Could you check a few things on this model? Use its own coordinates, in mm. A direction names the side the tool comes from. Coordinates: 2 decimals unless noted, no trailing zeros. Write each loop counter-clockwise with the first axis right and the second up, starting at its lowest first coordinate (ties: lowest second). Pieces come first, ordered by that corner, then holes.
Autodesk Inventor part; units mm, degrees
ref_plane "YZ Plane" through (0, 0, 0) normal (1, 0, 0) x (0, 1, 0)
ref_plane "XZ Plane" through (0, 0, 0) normal (0, 1, 0) x (-1, 0, 0)
ref_plane "XY Plane" through (0, 0, 0) normal (0, 0, 1) x (1, 0, 0)
sketch "Boceto1" plane through (0, 0, 0) normal (0, 0, 1) x (1, 0, 0)
  line L0 (-350, 205) -> (350, 205)
  line L1 (350, 205) -> (350, -205)
  line L2 (350, -205) -> (-350, -205)
  line L3 (-350, -205) -> (-350, 205)
  line L4 (-350, 205) -> (350, -205) construction
  line L5 (350, 205) -> (-350, -205) construction
  point P0 (0, 0)
  dimension "d0" = 700
  dimension "d1" = 410
extrude "Placa1" add sketch "Boceto1" along normal blind 5
sketch "Boceto2" plane through (-345, -205, 0) normal (-1, 0, 0) x (0, -1, 0)
  line L0 (-385, 0) -> (-25, 0)
  line L1 (-25, 0) -> (-25, 25)
  line L2 (-25, 25) -> (-385, 25)
  line L3 (-385, 25) -> (-385, 0)
edge flange "Pestaña1" height 25 angle 90 thickness 5 bend radius 5 thickness toward (-1, 0, 0) relief straight relief width 5 relief depth 2.5 edges at (-350, 0, 5) wall of the first edge with corners at (-345, 180, 0) (-345, -180, 0) (-345, -180, 25) (-345, 180, 25)
bend "Doblez1"
corner "Esquina1"
sketch "Boceto3" plane through (345, 205, 0) normal (1, 0, 0) x (0, 1, 0)
  line L0 (-385, 0) -> (-25, 0)
  line L1 (-25, 0) -> (-25, 25)
  line L2 (-25, 25) -> (-385, 25)
  line L3 (-385, 25) -> (-385, 0)
edge flange "Pestaña2" height 25 angle 90 thickness 5 bend radius 5 thickness toward (1, 0, 0) relief straight relief width 5 relief depth 2.5 edges at (350, 0, 5) wall of the first edge with corners at (345, -180, 0) (345, 180, 0) (345, 180, 25) (345, -180, 25)
bend "Doblez2"
corner "Esquina2"
equation "\"d2\" = Thickness"
equation "\"d3\" = BendReliefWidth"
equation "\"d4\" = BendReliefDepth"
equation "\"d5\" = MinimumRemnant"
equation "\"d6\" = TransitionRadius"
equation "\"d10\" = BendRadius"
equation "\"d11\" = CornerReliefSize"
equation "\"d12\" = GapSize"
equation "\"d13\" = JacobiRadiusSize"
equation "\"d14\" = BendReliefWidth"
equation "\"d15\" = BendReliefDepth"
equation "\"d16\" = MinimumRemnant"
equation "\"d17\" = TransitionRadius"
equation "\"d21\" = BendRadius"
equation "\"d22\" = CornerReliefSize"
equation "\"d23\" = GapSize"
equation "\"d24\" = JacobiRadiusSize"
equation "\"BendRadius\" = Thickness"
equation "\"BendReliefWidth\" = Thickness"
equation "\"BendReliefDepth\" = 0.5 * Thickness"
equation "\"TransitionRadius\" = BendRadius"
equation "\"JacobiRadiusSize\" = BendRadius"
equation "\"GapSize\" = Thickness"
properties part number "Fondo"
1. Please list where these lines run through material, in increasing order: line 1 along X through (y, z) = (162.5, 12.5); line 2 along X through (y, z) = (45, 9); line 3 along Z through (x, y) = (37.5, -84.5).
Verdict:
line 1: x = -350 to -345, 345 to 350
line 2: x = -349.95 to -344.9, 344.9 to 349.95
line 3: z = 0 to 5
2. For pin 1 (2 mm diameter, centred on x = -211, y = -161.5, fed in from +Z); pin 2 (6 mm diameter, centred on x = -346, z = 12, fed in from +Y); pin 3 (1.5 mm diameter, centred on y = 181.5, z = 3, fed in from -X), each with a flat end and sliding along its axis, tell me the tip position at first contact or that it passes through.
Verdict:
pin 1: stops at z = 5
pin 2: stops at y = 180
pin 3: stops at x = -337.5
3. On a 3-axis mill with a long thin cutter (end or side, diameter ignored), from which of +Z, -Z, +X, -X, +Y, -Y can I reach the whole of each face in a straight line? I mean faces 1 (the face through (-350, -3, 18)), 2 (the face through (345.2, 180, 12.7)), 3 (the face through (-345.2, -180, 12.7)), 4 (the face through (-345, -3, 17)). Say none if no direction works.
Verdict:
face 1: +Z, -Z, -X, +Y, -Y
face 2: +Z, -Z, +X
face 3: +Z, -Z, -X
face 4: +Z, +Y, -Y
4. I want a section at A-A on z = 14. Please give me the cut outline in (x, y), plus the area to 3 significant figures.
Verdict:
outline: (-350, -180) - (-345, -180) - (-345, 180) - (-350, 180) - close; (345, -180) - (350, -180) - (350, 180) - (345, 180) - close
area: 3,600 mm2
5. I want a section at B-B on y = 157.5. Please give me the cut outline in (x, z).
Verdict:
outline: (-350, 10) arc R10 ccw to (-340, 0) - (340, 0) arc R10 ccw to (350, 10) - (350, 25) - (345, 25) - (345, 10) arc R5 cw to (340, 5) - (-340, 5) arc R5 cw to (-345, 10) - (-345, 25) - (-350, 25) - close
6. If we mould it in two halves opening along X, with no side actions, what happens to faces 5 (the face through (345, 3, 17)), 6 (the face through (350, 3, 18)), 7 (the face through (-5, 3, 0)), 8 (the face through (-5, 3, 5))? For each: pulls with the +X half, pulls with the -X half, needs draft (parallel to the pull), parting line crosses it, or undercut.
Verdict:
face 5: undercut
face 6: pulls with the +X half
face 7: needs draft
face 8: undercut
7. I want a section at C-C on x = -77.5. Please give me the cut outline in (y, z), plus the area to 3 significant figures.
Verdict:
outline: (-205, 0) - (205, 0) - (205, 5) - (-205, 5) - close
area: 2,050 mm2
